Autodesk Inventor part; units mm, degrees
ref_plane "YZ Plane" through (0, 0, 0) normal (1, 0, 0) x (0, 1, 0)
ref_plane "XZ Plane" through (0, 0, 0) normal (0, 1, 0) x (-1, 0, 0)
ref_plane "XY Plane" through (0, 0, 0) normal (0, 0, 1) x (1, 0, 0)
sketch "スケッチ1" plane through (0, 0, 0) normal (1, 0, 0) x (0, 1, 0)
  circle A0 centre (0, 0) radius 13.5
  dimension "d0" = 27
extrude "押し出し1" add sketch "スケッチ1" along normal blind 15
sketch "スケッチ2" plane through (15, 0, 0) normal (1, 0, 0) x (0, 0, -1)
  circle A0 centre (0, 0) radius 11
  dimension "d3" = 22
extrude "押し出し2" add sketch "スケッチ2" along normal blind 140
sketch "スケッチ3" plane through (155, 0, 0) normal (1, 0, 0) x (0, 0, -1)
  circle A0 centre (0, 0) radius 13
  dimension "d6" = 26
extrude "押し出し3" add sketch "スケッチ3" along normal blind 15
sketch "スケッチ4" plane through (170, 0, 0) normal (1, 0, 0) x (0, 0, -1)
  circle A0 centre (0, 0) radius 11
  dimension "d9" = 22
extrude "押し出し4" add sketch "スケッチ4" along normal blind 12
thread "ねじ1"
sketch "スケッチ5" plane through (0, 0, 0) normal (-1, 0, 0) x (0, 0, 1)
  circle A0 centre (0, 0) radius 11
  line L0 (7.5498, 8) -> (-7.5498, 8)
  line L1 (0, 0) -> (-11, 0)
  line L2 (7.5498, -8) -> (-7.5498, -8)
  dimension "d14" = 22
  dimension "d15" = 8
extrude "押し出し5" add sketch "スケッチ5" along normal blind 21 contours A0 L2 L0
thread "ねじ2"
sketch "スケッチ6" plane through (0, 8, 7.5498) normal (0, 1, 0) x (1, 0, 0)
  circle A0 centre (-12, 7.5498) radius 6.5
  line L0 (-21, 0) -> (-21, 15.0997)
  line L1 (-21, 7.5498) -> (0, 7.5498)
  dimension "d20" = 13
  dimension "d21" = 0
  dimension "d22" = 9
extrude "押し出し6" cut sketch "スケッチ6" against normal through all
sketch "スケッチ7" plane through (182, 0, 0) normal (1, 0, 0) x (0, 0, -1)
  circle A0 centre (0, 0) radius 5
  dimension "d25" = 10
extrude "押し出し7" cut sketch "スケッチ7" against normal blind 100
properties part number "aircilinder_100_under" material "アルミニウム 6061"
Work out the finished part from the listing and answer in its coordinate system (mm). A direction names the side the tool comes from. Coordinates: 2 decimals unless noted, no trailing zeros. Write each loop counter-clockwise with the first axis right and the second up, starting at its lowest first coordinate (ties: lowest second). Pieces come first, ordered by that corner, then holes.
Q1. A cutting plane is placed at B-B, the plane y = 0. Give the vertices of the cut face in (x, z).
Q2. Find the intervals of material crossed by line 1 (X direction, y = 1.25, z = -11.75); line 2 (Y direction, x = 152, z = 0); line 3 (Y direction, x = 156.5, z = 0), in increasing order.
Q3. A cutting plane is placed at C-C, the plane x = 38. Give the vertices of the cut face in (y, z), then the cut area to 3 significant figures.
Q4. Which of the six approach directions +Z, -Z, +X, -X, +Y, -Y give full straight-line access (tool end or side, diameter ignored) to faces 1 (the face through (-6, 8, 3)), 2 (the face through (-10, 0, 11)), 3 (the face through (-6, -8, 3)), 4 (the face through (175.92, 10.74, 2.38)), 5 (the face through (15, -5, -10))?
Q5. A cutting plane is placed at A-A, the plane z = 0. Give the vertices of the cut face in (x, y).
Q6. Each of these flat-tipped pins is pushed along its axis until it touches: pin 1 Ø4.5 at (x, z) = (-7, 3.5) entering from -Y; pin 2 Ø1 at (x, z) = (29.5, 7) entering from +Y; pin 3 Ø1 at (x, z) = (150.5, -10) entering from +Y. Where does it stop, or does it pass through?
Q7. Determine the mould class of faces 6 (the face through (-10, 0, -11)), 7 (the face through (132.7, -4.88, 1.08)), 8 (the face through (-21, 0, 0)), 9 (the face through (162.395, 7.91, 10.316)) for opening direction Z: released by +Z, released by -Z, zero draft, split by the parting line, or undercut.
Findings below:
1. outline: (-21, -11) - (0, -11) - (0, -13.5) - (15, -13.5) - (15, -11) - (155, -11) - (155, -13) - (170, -13) - (170, -11) - (182, -11) - (182, -5) - (82, -5) - (82, 5) - (182, 5) - (182, 11) - (170, 11) - (170, 13) - (155, 13) - (155, 11) - (15, 11) - (15, 13.5) - (0, 13.5) - (0, 11) - (-21, 11) - close; hole circle Ø13 at (-12, 0)
2. line 1: x = 0 to 15, 155 to 170
2. line 2: y = -11 to -5, 5 to 11
2. line 3: y = -13 to -5, 5 to 13
3. outline: circle Ø22 at (0, 0)
3. area: 380 mm2
4. face 1: +Z, -Z, -X, +Y
4. face 2: +Z, -X
4. face 3: +Z, -Z, -X, -Y
4. face 4: +X
4. face 5: none
5. outline: (-21, -8) - (-18.5, -8) - (-18.5, 8) - (-21, 8) - close; (-5.5, -8) - (0, -8) - (0, -13.5) - (15, -13.5) - (15, -11) - (155, -11) - (155, -13) - (170, -13) - (170, -11) - (182, -11) - (182, -5) - (82, -5) - (82, 5) - (182, 5) - (182, 11) - (170, 11) - (170, 13) - (155, 13) - (155, 11) - (15, 11) - (15, 13.5) - (0, 13.5) - (0, 8) - (-5.5, 8) - close
6. pin 1: stops at y = -8
6. pin 2: stops at y = 8.87
6. pin 3: stops at y = 5.55
7. face 6: released by -Z
7. face 7: undercut
7. face 8: zero draft
7. face 9: split by the parting line
